The listing builds one solid part. Answer for the finished solid, in the listing's coordinates (mm). A direction names the side the tool comes from. Round coordinates to 2 decimals unless told otherwise and drop trailing zeros. Loops run counter-clockwise (first coordinate to the right, second up) from the corner with the lowest first, then second, coordinate; pieces in that order, holes last. Notation, with made-up numbers: (69, 23.25) -> (100, 23.25) arc R6 cw to (100, 31.25) -> close; hole circle Ø11 at (27, 76). An arc over 180 degrees is marked (long way). Write each question's results on one line, items separated by ' | '. Start each with the question number.
(1) The part is cut by section A-A (x = 149.35). Determine the outline of the cut face in (y, z).
(2) Straight lines are drawn through the part: probe 1 along X at (y, z) = (2.75, -10) (3 decimals); probe 2 along X at (y, z) = (3.25, -57.82); probe 3 along Z at (x, y) = (134.5, 4). For each, find the intervals that lie inside material, in ascending order.
(3) Flat-ended cylindrical pins translate along their axes: pin 1 (4 mm diameter, centred on x = 154.85, z = -96.51, fed in from -Y) (3 decimals); pin 2 (6.5 mm diameter, centred on y = 2, z = -26.5, fed in from -X). Find the tip coordinate at first contact, or state that the pin passes through.
(4) Determine the mould class of faces 4 (the face through (169, 0, -20)), 5 (the face through (136, 0, -26)), 6 (the face through (88, -6.35, -70)) for opening direction Z: released by +Z, released by -Z, zero draft, split by the parting line, or undercut.
(5) For faces 1 (the face through (159.35, 0, -10)), 2 (the face through (43.43, -0.09, -102.82)), 3 (the face through (8, 0, -33)), determine the directions among +Z, -Z, +X, -X, +Y, -Y from which every point of the face is accessible in a straight line to the end or side of a thin tool.
(6) The part is cut by section B-B (z = -10). Determine the outline of the cut face in (x, y) (3 decimals), plus the area to 3 significant figures.
(7) The part is cut by section D-D (z = -57.82). Determine the outline of the cut face in (x, y), plus the area to 3 significant figures.
(8) The part is cut by section C-C (y = -1.5). Count the separate pieces of the cut face and the enclosed holes in it, plus the area to 3 significant figures.
```python
from build123d import *

# Parameters (mm, degrees)
SKETCH1_R           = 2.5
SKETCH1_W           = 22
SKETCH1_H           = 13
BOSS_EXTRUDE1_DEPTH = 6.35


with BuildPart() as part:
    # Sketch1 → Boss-Extrude1 (new, symmetric)
    with BuildSketch(Plane(origin=(0, 0, 0), x_dir=(1, 0, 0), z_dir=(0, 1, 0))):
        Polygon((0, 0), (159.35, 0), (159.35, 20), (179.35, 20), (179.35, 112.82), (0, 112.82), (0, 33), (16, 33), (16, 20), (0, 20), align=None)
        with Locations(Location((43.48717527, 57.82, 0), (0, 0, 270))):
            Circle(SKETCH1_R, mode=Mode.SUBTRACT)
        with Locations(Location((88.86282473, 57.82, 0), (0, 0, 270))):
            Circle(SKETCH1_R, mode=Mode.SUBTRACT)
        with Locations(Location((131.86282473, 57.82, 0), (0, 0, 270))):
            Circle(SKETCH1_R, mode=Mode.SUBTRACT)
        with Locations(Location((154.85, 96.505782571, 0), (0, 0, 270))):
            Circle(SKETCH1_R, mode=Mode.SUBTRACT)
        with Locations(Location((10, 10, 0), (0, 0, 270))):
            Circle(SKETCH1_R, mode=Mode.SUBTRACT)
        with Locations(Location((79.675, 10, 0), (0, 0, 270))):
            Circle(SKETCH1_R, mode=Mode.SUBTRACT)
        with Locations(Location((149.35, 10, 0), (0, 0, 270))):
            Circle(SKETCH1_R, mode=Mode.SUBTRACT)
        with BuildLine():
            Line((40.98717527, 95.32), (40.98717527, 100.32))
            ThreePointArc((40.98717527, 100.32), (43.48717527, 102.82), (45.98717527, 100.32))
            Line((45.98717527, 100.32), (45.98717527, 95.32))
            ThreePointArc((45.98717527, 95.32), (43.48717527, 92.82), (40.98717527, 95.32))
        make_face(mode=Mode.SUBTRACT)
        with Locations((125, 26.5)):
            Rectangle(SKETCH1_W, SKETCH1_H, mode=Mode.SUBTRACT)
    extrude(amount=BOSS_EXTRUDE1_DEPTH, both=True)


solid = part.part
```
Checked values:
1) outline: (-6.35, -112.82) -> (6.35, -112.82) -> (6.35, -12.5) -> (-6.35, -12.5) -> close; (-6.35, -7.5) -> (6.35, -7.5) -> (6.35, 0) -> (-6.35, 0) -> close
2) probe 1: x = 0 to 7.5, 12.5 to 77.175, 82.175 to 146.85, 151.85 to 159.35 | probe 2: x = 0 to 40.99, 45.99 to 86.36, 91.36 to 129.36, 134.36 to 179.35 | probe 3: z = -112.82 to -33, -20 to 0
3) pin 1: passes through | pin 2: stops at x = 16
4) face 4: released by +Z | face 5: undercut | face 6: zero draft
5) face 1: +Z, +X, +Y, -Y | face 2: +Y, -Y | face 3: -X, +Y, -Y
6) outline: (0, -6.35) -> (7.5, -6.35) -> (7.5, 6.35) -> (0, 6.35) -> close; (12.5, -6.35) -> (77.175, -6.35) -> (77.175, 6.35) -> (12.5, 6.35) -> close; (82.175, -6.35) -> (146.85, -6.35) -> (146.85, 6.35) -> (82.175, 6.35) -> close; (151.85, -6.35) -> (159.35, -6.35) -> (159.35, 6.35) -> (151.85, 6.35) -> close | area: 1,830 mm2
7) outline: (0, -6.35) -> (40.99, -6.35) -> (40.99, 6.35) -> (0, 6.35) -> close; (45.99, -6.35) -> (86.36, -6.35) -> (86.36, 6.35) -> (45.99, 6.35) -> close; (91.36, -6.35) -> (129.36, -6.35) -> (129.36, 6.35) -> (91.36, 6.35) -> close; (134.36, -6.35) -> (179.35, -6.35) -> (179.35, 6.35) -> (134.36, 6.35) -> close | area: 2,090 mm2
8) separate pieces: 1 | enclosed holes: 9 | area: 19,200 mm2
